Geometry check sheet. Reference: drawing and pictorial views, mm from the part's lowest x, y, z. A direction names the side the tool comes from. Give positions to 0.01 mm unless a question says otherwise; leave off trailing zeros. Order: outer loops, then holes, each group sorted by start corner. A loop starts at its lowest first (then second) coordinate and runs counter-clockwise, first axis right, second up. Notation, with made-up numbers: (75, -8.5) - (126, -8.5) arc R19 ccw to (126, 27.5) - close; hole circle Ø9 at (-30, 9). An arc over 180 degrees is marked (long way). Answer in a Markdown table with one row per item.
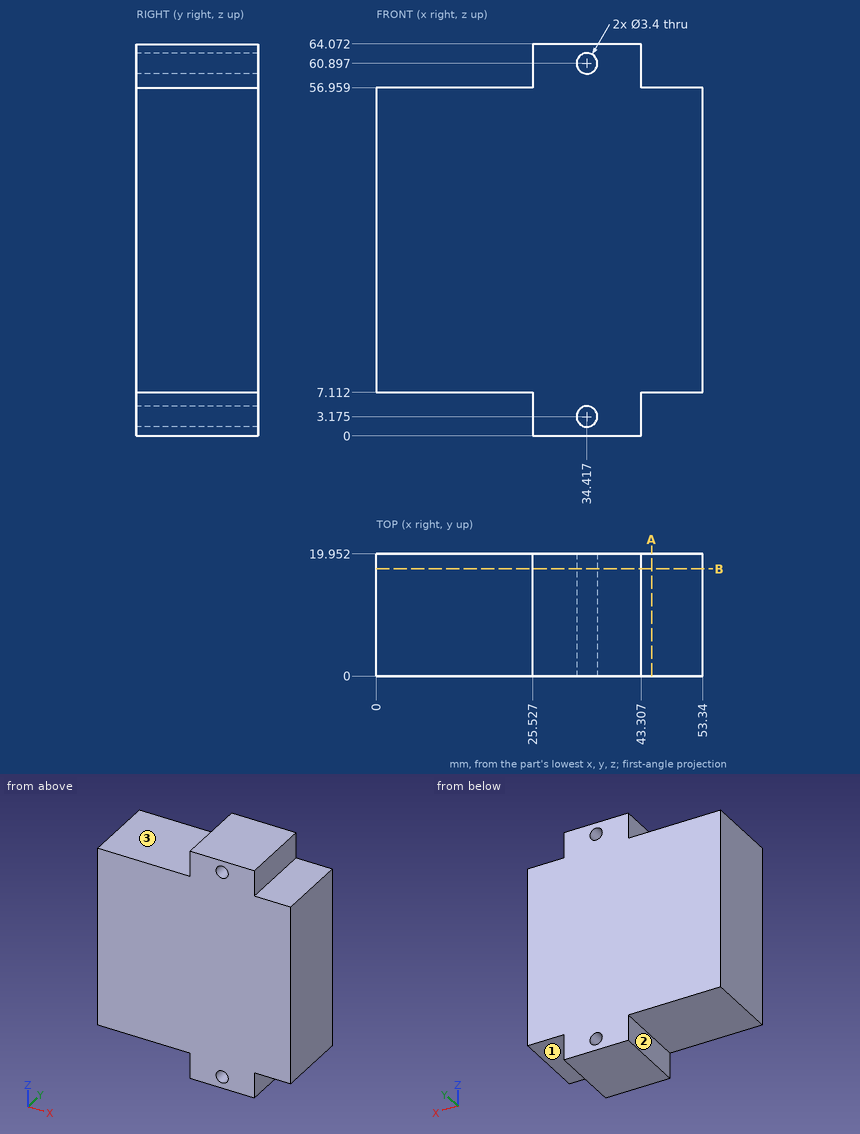
(1) Access from +Z, -Z, +X, -X, +Y, -Y to the whole of each face (thin tool, end or side, straight path). Record for the marked faces 1, 2 and 3.
Geometry says:
| item | result |
|---|---|
| face 1 | -Z, +X, +Y, -Y |
| face 2 | -Z, -X, +Y, -Y |
| face 3 | +Z, -X, +Y, -Y |
(2) Cross-section at B-B, the plane y = 17.5. Record the cut outline in (x, z) (1 decimal), then the cut area to 3 significant figures.
Geometry says:
| item | result |
|---|---|
| outline | (0, 7.1) - (25.5, 7.1) - (25.5, 0) - (43.3, 0) - (43.3, 7.1) - (53.3, 7.1) - (53.3, 57) - (43.3, 57) - (43.3, 64.1) - (25.5, 64.1) - (25.5, 57) - (0, 57) - close; hole circle Ø3.4 at (34.4, 3.2); hole circle Ø3.4 at (34.4, 60.9) |
| area | 2,890 mm² |
(3) Cross-section at A-A, the plane x = 45. Record the cut outline in (y, z).
Geometry says:
| item | result |
|---|---|
| outline | (0, 7.11) - (19.95, 7.11) - (19.95, 56.96) - (0, 56.96) - close |
(4) Gauge pin test, flat ends, axial feed: P1, Ø3.5, axis at y = 5.5, z = 3.5, coming from the -X side; P2, Ø5, axis at x = 49, y = 5.5, coming from the -Z side; P3, Ø5, axis at x = 50, y = 7.5, coming from the +Z side. Record the tip position at first contact, or that the pin passes through.
Geometry says:
| item | result |
|---|---|
| P1 | x = 25.53 |
| P2 | z = 7.11 |
| P3 | z = 56.96 |
(5) Thickness scan on L1, parallel to Z at x = 34, y = 17 (1 decimal); L2, parallel to Z at x = 11, y = 12.75; L3, parallel to X at y = 5.5, z = 5.5. Record the ranges inside material, lowest first.
Geometry says:
| item | result |
|---|---|
| L1 | 0 to 1.5, 4.8 to 59.2, 62.5 to 64.1 |
| L2 | 7.11 to 56.96 |
| L3 | 25.53 to 43.31 |
